CAD build for the part. Positions are in the model's coordinates, mm. Face numbers are marked on the shaded views. A direction names the side the tool comes from. Round coordinates to 2 decimals unless told otherwise and drop trailing zeros. Order: outer loops, then holes, each group sorted by start corner. A loop starts at its lowest first (then second) coordinate and runs counter-clockwise, first axis right, second up. Notation, with made-up numbers: (39.5, 55.25) -> (47.5, 55.25) arc R32 ccw to (47.5, 91.25) -> close; hole circle Ø7 at (-17.5, 40.5). An arc over 180 degrees is marked (long way). Answer as CSV lines item,"result". Start each with the question number.
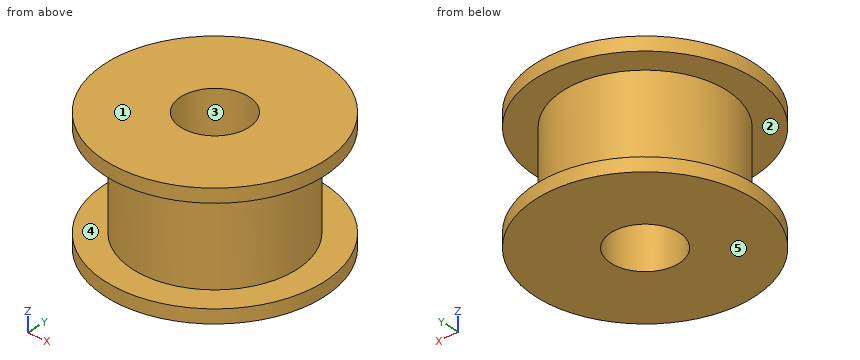
from build123d import *

# Parameters (mm, degrees)
SKETCH3_R           = 8
BOSS_EXTRUDE1_DEPTH = 4.5
SKETCH4_R           = 2.5
CUT_EXTRUDE1_DEPTH  = 15.456832295
SKETCH6_R           = 8
SKETCH6_R_2         = 6
CUT_EXTRUDE2_DEPTH  = 3.5


with BuildPart() as part:
    # Sketch3 → Boss-Extrude1 (new, symmetric)
    with BuildSketch(Plane.XY):
        Circle(SKETCH3_R)
    extrude(amount=BOSS_EXTRUDE1_DEPTH, both=True)

    # Sketch4 → Cut-Extrude1 (cut, through all)
    with BuildSketch(Plane(origin=(0, 0, -4.5), x_dir=(-1, 0, 0), z_dir=(0, 0, -1))):
        Circle(SKETCH4_R)
    extrude(amount=-CUT_EXTRUDE1_DEPTH, mode=Mode.SUBTRACT)

    # Sketch6 → Cut-Extrude2 (cut, symmetric)
    with BuildSketch(Plane.XY):
        Circle(SKETCH6_R)
        Circle(SKETCH6_R_2, mode=Mode.SUBTRACT)
    extrude(amount=CUT_EXTRUDE2_DEPTH, both=True, mode=Mode.SUBTRACT)


solid = part.part
Item 1: Pin check, flat tips, straight feed: pin 1 (1 mm diameter, centred on x = 1, z = 0.5, fed in from +Y); pin 2 (1.5 mm diameter, centred on y = -5.5, z = -1, fed in from -X); pin 3 (3 mm diameter, centred on y = 3, z = 3, fed in from -X). Stop position of each tip, or through.
Item 2: Band-saw the part on A-A, the plane x = 0. Give the cut face in (y, z), and give its area (3 significant figures).
Item 3: Band-saw the part on C-C, the plane z = 0. Give the cut face in (x, y).
Item 4: Mould opens along Z. For the marked faces 1, 2 and 3 say: released by +Z, released by -Z, zero draft, split by the parting line, or undercut.
Item 5: Band-saw the part on D-D, the plane x = 2.75. Give the cut face in (y, z), and give its area (3 significant figures).
Item 6: Tool access for the marked faces 4 and 5: list every direction of +Z, -Z, +X, -X, +Y, -Y with a clear straight run to the whole face (end or side of a thin tool).
Item 7: Probe line 1 (Y direction, x = 0, z = 0.5); line 2 (Z direction, x = 5, y = -4.25); line 3 (X direction, y = -1.25, z = 0.25). List the from-to ranges inside material, lowest first.
Values:
1,pin 1,"y = 5.98"
1,pin 2,"x = -3.67"
1,pin 3,"x = -7.84"
2,outline,"(-8, -4.5) -> (-2.5, -4.5) -> (-2.5, 4.5) -> (-8, 4.5) -> (-8, 3.5) -> (-6, 3.5) -> (-6, -3.5) -> (-8, -3.5) -> close; (2.5, -4.5) -> (8, -4.5) -> (8, -3.5) -> (6, -3.5) -> (6, 3.5) -> (8, 3.5) -> (8, 4.5) -> (2.5, 4.5) -> close"
2,area,"71.0 mm²"
3,outline,"circle Ø12 at (0, 0); hole circle Ø5 at (0, 0)"
4,face 1,"released by +Z"
4,face 2,"undercut"
4,face 3,"zero draft"
5,outline,"(-7.51, -4.5) -> (7.51, -4.5) -> (7.51, -3.5) -> (5.33, -3.5) -> (5.33, 3.5) -> (7.51, 3.5) -> (7.51, 4.5) -> (-7.51, 4.5) -> (-7.51, 3.5) -> (-5.33, 3.5) -> (-5.33, -3.5) -> (-7.51, -3.5) -> close"
5,area,"105 mm²"
6,face 4,"none"
6,face 5,"-Z, +X, -X, +Y, -Y"
7,line 1,"-6 to -2.5, 2.5 to 6"
7,line 2,"-4.5 to -3.5, 3.5 to 4.5"
7,line 3,"-5.87 to -2.17, 2.17 to 5.87"
